Input: part model. Units: mm. Frame: model coordinates. Face numbers are marked on the shaded views. A direction names the side the tool comes from. Round coordinates to 2 decimals unless told otherwise and drop trailing zeros. Loops run counter-clockwise (first coordinate to the right, second up) from the corner with the lowest first, then second, coordinate; pieces in that order, holes last.
1) Draft query along Y for the marked faces 1, 2, 3 and 4. Return one class per face: pulls with the +Y half, pulls with the -Y half, needs draft (parallel to the pull), parting line crosses it, or undercut.
2) Access query for the marked faces 5, 6, 7 and 8. Directions: +Z, -Z, +X, -X, +Y, -Y. A direction counts if a zero-diameter tool reaches every point of the face in a straight line with its end or side. Return the directions, or none.
3) Ray query, line 1 along Y through (x, z) = (-32, 5.5); line 2 along X through (y, z) = (46, 1.25); line 3 along Y through (x, z) = (-27.5, 5.75). Return the intervals inside material, ascending.
4) Section B-B, the plane y = 8.5. Return loops of the section in (x, z), and give its area (3 significant figures).
5) Section A-A, the plane x = -41. Return loops of the section in (y, z), and give its area (3 significant figures).
6) Section C-C, the plane z = 2.25. State how many separate pieces and enclosed holes the cut face has, and give its area (3 significant figures).
7) First-contact query: pin 1 (1 mm diameter, centred on x = -46.5, z = 3.5, fed in from -Y) (3 decimals); pin 2 (1.9 mm diameter, centred on x = -29.5, z = 2.5, fed in from +Y); pin 3 (1.9 mm diameter, centred on y = 47, z = 4.5, fed in from -X). Flat tips, straight axial feed; report the tip coordinate or a pass-through.
from build123d import *

# Parameters (mm, degrees)
F1_DEPTH = 6.35
F3_D     = 3.3
F4_R     = 2.99974
F5_W     = 17.2659438103
F5_H     = 5.7261204347
F6_DEPTH = 6.35
F8_D     = 3.3
F10_D    = 3.3


with BuildPart() as f1:
    # F0 (on Top) → F1 (new body)
    with BuildSketch(Plane.XY):
        Polygon((-40.1544658885, 51.4584925147), (-49.2730658885, 51.4584925147), (-49.2730658885, 19.7084925147), (-19.3046238273, 19.7084925147), (-16.1006658885, 45.0133569539), (-16.1006658885, 51.4584925147), (-24.9906658885, 51.4584925147), (-24.9906658885, 45.0133569539), (-40.1544658885, 45.0133569539), align=None)
    extrude(amount=F1_DEPTH)

    # F3 (through all)
    with Locations(Plane.YZ.offset(-16.1006658885)):
        with Locations((48.2228761828, 3.1560653739)):
            Hole(F3_D / 2)

    # F4
    f4_edges = [f1.edges().sort_by_distance(p)[0] for p in [
        (-20.545666, 51.458493, 0),
        (-20.545666, 51.458493, 6.35),
        (-44.713766, 51.458493, 0),
        (-44.713766, 51.458493, 6.35),
    ]]
    fillet(f4_edges, radius=F4_R)

    # F5 (on Top) → F6 (join)
    with BuildSketch(Plane.XY):
        with BuildLine():
            Line((-48.0508575901, -9.525), (-44.8758575901, -9.525))
            Line((-44.8758575901, -9.525), (-44.8758575901, -1.5875))
            ThreePointArc((-44.8758575901, -1.5875), (-44.4108896053, -0.4649679849), (-43.2883575901, 0))
            Line((-43.2883575901, 0), (-31.6287431982, 0))
            ThreePointArc((-31.6287431982, 0), (-30.5254053426, -0.4511271755), (-30.0542057782, -1.54604321))
            Line((-30.0542057782, -1.54604321), (-29.9068968743, -9.6117341891))
            Line((-29.9068968743, -9.6117341891), (-23.7938760812, -9.5000881572))
            ThreePointArc((-23.7938760812, -9.5000881572), (-22.7076296204, -9.03764911), (-22.248025792, -7.9502))
            Line((-22.248025792, -7.9502), (-19.3092767149, 19.7430392682))
            Line((-19.3092767149, 19.7430392682), (-49.2723993957, 19.7069626302))
            Line((-49.2723993957, 19.7069626302), (-49.6256575901, -7.9502))
            ThreePointArc((-49.6256575901, -7.9502), (-49.1644093491, -9.063751759), (-48.0508575901, -9.525))
        make_face()
        with Locations((-33.5407005623, 15.7169797458)):
            Rectangle(F5_W, F5_H, mode=Mode.SUBTRACT)
    extrude(amount=F6_DEPTH)

    # F8 (through all)
    with Locations(Plane(origin=(-49.516033415, 0.6324562209, 0), x_dir=(-0.0127717144, -0.9999184383, 0), z_dir=(-0.9999184383, 0.0127717144, 0))):
        with Locations((5.4090460762, 3.175)):
            Hole(F8_D / 2)

    # F10 (through all)
    with Locations(Plane(origin=(-49.516033415, 0.6324562209, 0), x_dir=(-0.0127717144, -0.9999184383, 0), z_dir=(-0.9999184383, 0.0127717144, 0))):
        with Locations((-14.6038243547, 3.1806000043)):
            Hole(F10_D / 2)


solid = f1.part
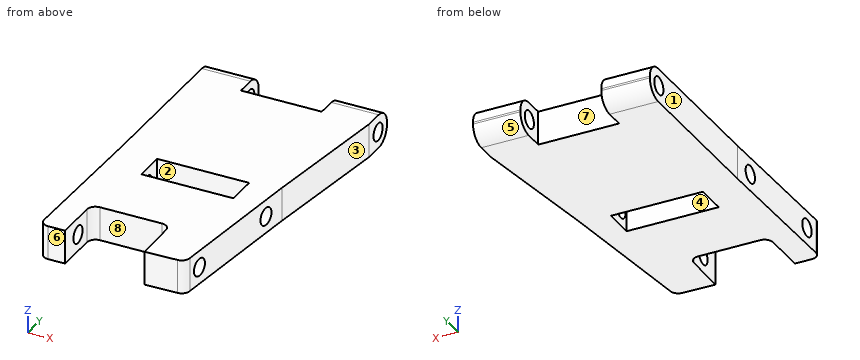
Final values:
1. face 1: needs draft
1. face 2: undercut
1. face 3: pulls with the -Y half
1. face 4: undercut
2. face 5: -Z, +X, -X, +Y
2. face 6: +Z, -Z, -X, -Y
2. face 7: +Z, -Z, +Y
2. face 8: +Z, -Z, -Y
3. line 1: y = 0 to 12.85, 18.58 to 45.01
3. line 2: x = -49.27 to -40.15, -24.99 to -16.1
3. line 3: y = -9.57 to 12.85, 18.58 to 45.01
4. outline: (-49.42, 0) - (-20.5, 0) - (-20.5, 6.35) - (-49.42, 6.35) - close
4. area: 184 mm2
5. outline: (0, 0) - (12.85, 0) - (12.85, 6.35) - (0, 6.35) - close; (18.58, 0) - (48.46, 0) arc R3 ccw to (51.46, 3) - (51.46, 3.35) arc R3 ccw to (48.46, 6.35) - (18.58, 6.35) - close; hole circle Ø3.3 at (48.22, 3.16)
5. area: 278 mm2
6. separate pieces: 6
6. enclosed holes: 0
6. area: 1,390 mm2
7. pin 1: stops at y = -9.525
7. pin 2: stops at y = 45.01
7. pin 3: stops at x = -49.27
